CAD build for the part. Positions are in the model's coordinates, mm. Round coordinates to 2 decimals unless told otherwise and drop trailing zeros. Order: outer loops, then holes, each group sorted by start corner. A loop starts at its lowest first (then second) coordinate and runs counter-clockwise, first axis right, second up. Notation, with made-up numbers: (-23.75, 19) - (6.25, 19) arc R16 cw to (6.25, 28) - close; hole circle Ø10 at (23, -32). An arc over 180 degrees is marked (long way). Write item = value, one per line.
from build123d import *

# Parameters (mm, degrees)
F0_R      = 13.5
F1_DEPTH  = 0.024
F3_R      = 10
F1_FACE_R = 13.5


with BuildPart() as f1:
    # F0 (on Front) → F1 (new body)
    with BuildSketch(Plane.XZ):
        Circle(F0_R)
    extrude(amount=F1_DEPTH)

    # F3 (on offset) → F4 section 0
    with BuildSketch(Plane.XZ.offset(11)):
        Circle(F3_R)
    # F1_face (on face) → F4 section 1
    with BuildSketch(Plane.XZ.offset(0.024)):
        Circle(F1_FACE_R)
    loft()

    # F5: F1 across plane


with BuildPart() as f1_1:
    add(f1.part)
    add(f1.part.mirror(Plane.XZ))


solid = f1_1.part
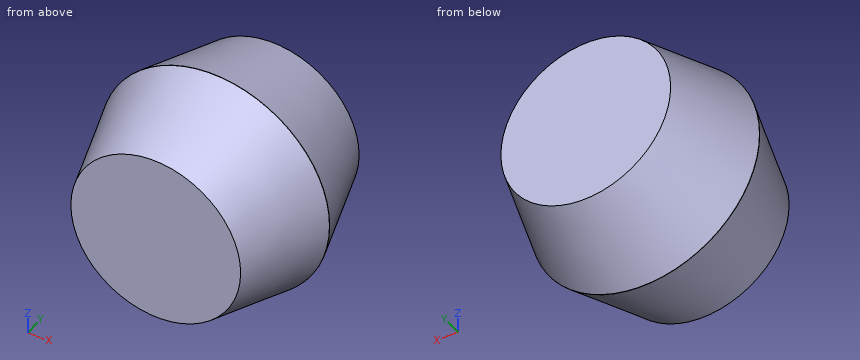
(1) Band-saw the part on A-A on x = 0. List the corners of the cut face in (y, z), plus the area to 3 significant figures.
Solved:
outline = (-11, -10) - (-0.02, -13.5) - (0.02, -13.5) - (11, -10) - (11, 10) - (0.02, 13.5) - (-0.02, 13.5) - (-11, 10) - close
area = 517 mm²
(2) Drop flat-ended pins along their axis: pin 1 (1 mm diameter, centred on x = 10, y = -8, fed in from +Z); pin 2 (5 mm diameter, centred on x = -5, y = -3.5, fed in from -Z); pin 3 (8 mm diameter, centred on y = 8, z = 2.5, fed in from +X). Give the stop position or say it passes through.
Solved:
pin_1 = 5.52
pin_2 = -12.55
pin_3 = 12.1
(3) Band-saw the part on C-C on y = 6. List the corners of the cut face in (x, z), plus the area to 3 significant figures.
Solved:
outline = circle Ø23.19 at (0, 0)
area = 422 mm²
(4) Probe line 1 along X through (y, z) = (1.25, 11.75); line 2 along Z through (x, y) = (-3, -1.25); line 3 along Z through (x, y) = (-9, 5.25). List the from-to ranges inside material, lowest first.
Solved:
line_1 = -5.81 to 5.81
line_2 = -12.76 to 12.76
line_3 = -7.68 to 7.68
(5) Band-saw the part on B-B on y = -2.75. List the corners of the cut face in (x, z), plus the area to 3 significant figures.
Solved:
outline = circle Ø25.26 at (0, 0)
area = 501 mm²
